Autodesk Inventor part; units mm, degrees
ref_plane "YZ Plane" through (0, 0, 0) normal (1, 0, 0) x (0, 1, 0)
ref_plane "XZ Plane" through (0, 0, 0) normal (0, 1, 0) x (-1, 0, 0)
ref_plane "XY Plane" through (0, 0, 0) normal (0, 0, 1) x (1, 0, 0)
sketch "Sketch1" plane through (0, 0, 0) normal (0, 1, 0) x (-1, 0, 0)
  line L0 (7, 100) -> (-7, 100)
  line L1 (-7, 100) -> (-7, -100)
  line L2 (-7, -100) -> (7, -100)
  line L3 (7, -100) -> (7, 100)
  point P0 (0, 0)
  point P1 (7, 0)
  point P2 (0, 100)
  dimension "d0" = 14
  dimension "d1" = 200
extrude "Extrusion1" add sketch "Sketch1" along normal blind 5.334
sketch "Sketch2" plane through (0, 5.334, 0) normal (0, 1, 0) x (1, 0, 0)
  line L0 (-7, -92) -> (1, -92)
  line L1 (1, -92) -> (1, 92)
  line L2 (1, 92) -> (-7, 92)
  line L3 (-7, 92) -> (-7, -92)
  line L4 (-7, 100) -> (-7, -100)
  line L5 (7, -100) -> (7, 100)
  line L6 (-7, -100) -> (7, -100)
  line L7 (7, 100) -> (-7, 100)
  point P0 (0, 0)
  point P1 (-7, 0)
  dimension "d4" = 6
  dimension "d5" = 8
  dimension "d6" = 8
extrude "Extrusion2" cut sketch "Sketch2" against normal through all contours L3 L2 L1 L0
sketch "Sketch3" plane through (-7, 0, 100) normal (0, 0, 1) x (1, 0, 0)
  line L0 (0, 0) -> (6, 0)
  line L1 (6, 0) -> (6, 5.334)
  line L2 (6, 5.334) -> (0, 5.334)
  line L3 (0, 5.334) -> (0, 0)
  line L4 (0, 5.334) -> (14, 5.334)
  point P0 (7, 0)
  point P1 (7, 5.334)
  dimension "d9" = 6
extrude "Extrusion3" add sketch "Sketch3" along normal blind 5.334
sketch "Sketch4" plane through (7, 0, 100) normal (1, 0, 0) x (0, 0, -1)
  line L0 (0, 5.334) -> (200, 5.334)
  line L1 (0, 0) -> (200, 0)
  line L2 (8, 5.334) -> (14, 5.334)
  line L3 (14, 5.334) -> (14, 0)
  line L4 (14, 0) -> (8, 0)
  line L5 (8, 0) -> (8, 5.334)
  line L6 (0, 0) -> (0, 5.334)
  point P0 (100, 0)
  dimension "d13" = 8
  dimension "d14" = 6
extrude "Extrusion4" add sketch "Sketch4" along normal blind 5.334 contours L0 L3 L1 L5
pattern_linear "Rectangular Pattern1" count 3 spacing 25.4 along (0, 0, -1) of "Extrusion4"
mirror "Mirror1" about plane through (0, 0, 0) normal (0, 0, 1) of "Extrusion3", "Extrusion4", "Rectangular Pattern1"
fillet "Fillet2" radius 3.175 4 edges at (-7, 2.667, 92) (1, 2.667, 92) (-7, 2.667, -92) (1, 2.667, -92)
equation "\"d6\" = d5"
properties part number "base_support"
The model under review builds one solid part; all positions refer to its coordinate system, in mm. A direction names the side the tool comes from. Give positions to 0.01 mm unless a question says otherwise; leave off trailing zeros. Write each loop counter-clockwise with the first axis right and the second up, starting at its lowest first coordinate (ties: lowest second). Pieces come first, ordered by that corner, then holes.
1. For P1, Ø2.5, axis at y = 2.5, z = 95.5, coming from the +X side; P2, Ø1.5, axis at x = 10, y = 1.5, coming from the +Z side; P3, Ø3, axis at x = 7.5, y = 3, coming from the +Z side, all flat-tipped, find the tip position at first contact; note any pin that passes through.
2. Add section A-A, the plane z = -76. Write out the cut boundary in (x, y).
3. Add section B-B, the plane x = 3. Write out the cut boundary in (y, z), plus the area to 3 significant figures.
4. Draft analysis for pull direction Z (two halves, no side actions). For faces 1 (the flat face through (10, 3, 92)), 2 (the flat face through (10, 3, -86)), 3 (the flat face through (-7, 3, 100)), state which applies: +Z half, -Z half, draft (parallel to the pull), parting line (faces both ways), or undercut.
5. Tool access review of faces 4 (the flat face through (7, 3, -96)), 5 (the flat face through (7, 3, -51)), 6 (the cylindrical face through (0.09, 2.63, 91.05)): name each direction out of +Z, -Z, +X, -X, +Y, -Y from which nothing blocks a thin tool from reaching the whole face with its end or side.
6. Wall thickness on L1, parallel to Z at x = 8, y = 5; L2, parallel to X at y = 4.8, z = 44.5; L3, parallel to Z at x = -6, y = 3.15: over which ranges is each line inside the solid? List them lowest first.
Worked answers:
1. P1: stops at x = 7
1. P2: stops at z = 92
1. P3: stops at z = 100
2. outline: (1, 0) - (7, 0) - (7, 5.33) - (1, 5.33) - close
3. outline: (0, -100) - (5.33, -100) - (5.33, 100) - (0, 100) - close
3. area: 1,070 mm2
4. face 1: +Z half
4. face 2: undercut
4. face 3: draft
5. face 4: -Z, +X, +Y, -Y
5. face 5: +X, +Y, -Y
5. face 6: -X, +Y, -Y
6. L1: z = -92 to -86, -66.6 to -60.6, -41.2 to -35.2, 35.2 to 41.2, 60.6 to 66.6, 86 to 92
6. L2: x = 1 to 7
6. L3: z = -105.33 to -92.86, 92.86 to 105.33
